from build123d import *

# Parameters (mm, degrees)
F1_DEPTH = 5
F2_SIZE  = 0.5


# Not quite as in the source:
# - ends of sketch curves that miss each other by under 0.0002 mm in the source are joined


with BuildPart() as f1:
    # F0 (on Front) → F1 (new body)
    with BuildSketch(Plane.XZ):
        with BuildLine():
            Line((12.196068, 40.75), (-12.196068, 40.75))
            ThreePointArc((-12.196068, 40.75), (-17.5303965634, -0.7793616591), (-30, -40.75))
            Line((-30, -40.75), (30, -40.75))
            ThreePointArc((30, -40.75), (17.5303965634, -0.7793616591), (12.196068, 40.75))
        make_face()
    extrude(amount=F1_DEPTH)

    # F2
    f2_edges = [f1.edges().sort_by_distance(p)[0] for p in [
        (-17.530397, 0, -0.779362),
        (-17.530397, -5, -0.779362),
        (17.530397, -5, -0.779362),
        (17.530397, 0, -0.779362),
    ]]
    chamfer(f2_edges, length=F2_SIZE)


solid = f1.part
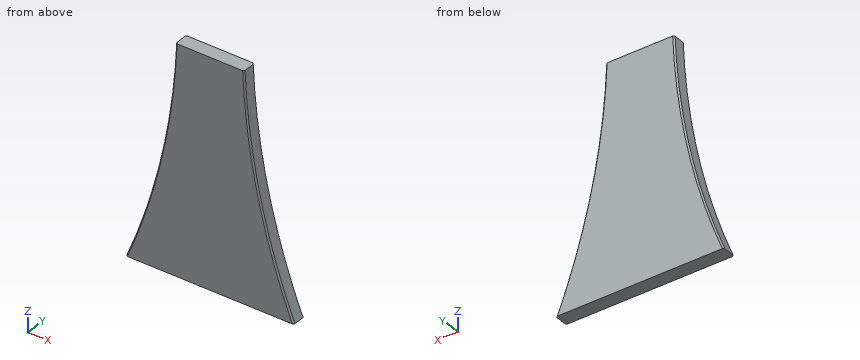
For this review, take the finished solid that the model builds, in its own axes (mm). Give positions to 0.01 mm unless a question says otherwise; leave off trailing zeros. Loops run counter-clockwise (first coordinate to the right, second up) from the corner with the lowest first, then second, coordinate; pieces in that order, holes last.
Item 1: Insertion check: pin 1 (3 mm diameter, centred on x = 17.5, z = 3, fed in from +Y). The pin has a flat end and moves straight along its axis. Give the tip position at first contact, or say it passes through.
Item 2: For line 1 along X through (y, z) = (-1.85, -2.5); line 2 along X through (y, z) = (-3.95, 12.5), list the stretches that pass through material, from the lowest coordinate up.
Item 3: Take a section at A-A, the plane y = -2.05. State the section outline as (x, z) points, and give its area (3 significant figures).
Calculated:
1. pin 1: stops at y = 0
2. line 1: x = -17.91 to 17.91
2. line 2: x = -15.02 to 15.02
3. outline: (-30, -40.75) - (30, -40.75) arc R240.04 cw to (12.2, 40.75) - (-12.2, 40.75) arc R240.04 cw to start
3. area: 3,030 mm2
